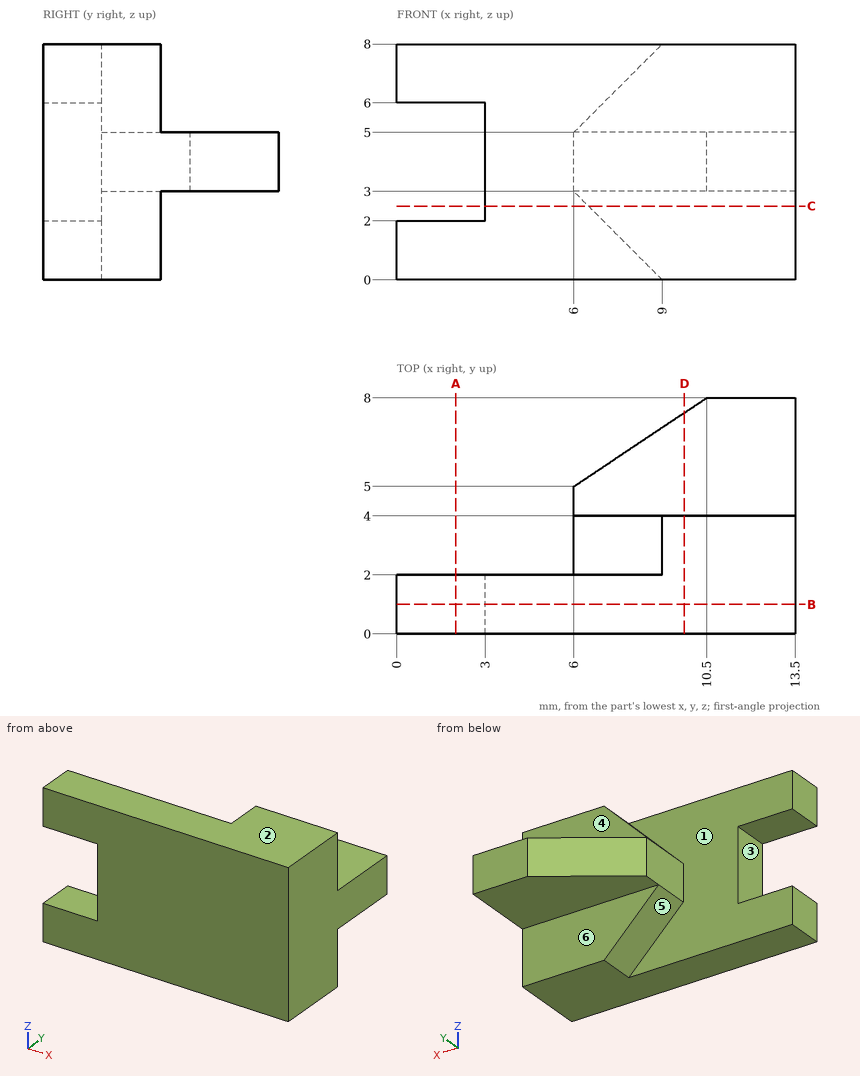
Check sheet for the drawn part. Datum: minimum x, y, z corner. Units: mm. A direction names the side the tool comes from. Give positions to 0.01 mm unless a question says otherwise; leave off trailing zeros. Order: outer loops, then holes, each group sorted by start corner. A loop starts at its lowest first (then second) coordinate and runs counter-clockwise, first axis right, second up. Notation, with made-up numbers: (-38, 68.25) -> (-25, 68.25) arc R29 ccw to (-25, 98.25) -> close; hole circle Ø7 at (85.5, 81). An arc over 180 degrees is marked (long way). One line per item, written item: value.
(1) Tool access check on the marked faces 4, 5 and 6. Record the directions out of +Z, -Z, +X, -X, +Y, -Y that give a thin tool (end or side, any length) a straight path to the whole face; none if there is none.
Final values:
face 4: +Z, +X, -X, +Y
face 5: -Z, -X, +Y
face 6: -Z, +X, -X, +Y
(2) Sectioned sample at A-A on x = 2. Record the cut outline in (y, z).
Final values:
outline: (0, 0) -> (2, 0) -> (2, 2) -> (0, 2) -> close; (0, 6) -> (2, 6) -> (2, 8) -> (0, 8) -> close
(3) Sectioned sample at C-C on z = 2.5. Record the cut outline in (x, y).
Final values:
outline: (3, 0) -> (13.5, 0) -> (13.5, 4) -> (6.5, 4) -> (6.5, 2) -> (3, 2) -> close
(4) Sectioned sample at D-D on x = 9.75. Record the cut outline in (y, z).
Final values:
outline: (0, 0) -> (4, 0) -> (4, 3) -> (7.5, 3) -> (7.5, 5) -> (4, 5) -> (4, 8) -> (0, 8) -> close
(5) Draft check along Z on the marked faces 1, 2 and 3. Enter one of: pulls with the +Z half, pulls with the -Z half, needs draft (parallel to the pull), parting line crosses it, or undercut.
Final values:
face 1: needs draft
face 2: pulls with the +Z half
face 3: undercut
(6) Gauge pin test, flat ends, axial feed: pin 1 (4 mm diameter, centred on x = 6, z = 2.5, fed in from +Y); pin 2 (2 mm diameter, centred on x = 5.5, y = 6, fed in from +Z); pin 3 (2.5 mm diameter, centred on x = 8, z = 6.5, fed in from +Y); pin 4 (0.6 mm diameter, centred on y = 1, z = 4, fed in from -X). Record the tip position at first contact, or that the pin passes through.
Final values:
pin 1: y = 6.29
pin 2: through
pin 3: y = 4
pin 4: x = 3
(7) Scan lines: line 1 along Z through (x, y) = (12.25, 6.5); line 2 along Y through (x, z) = (9.5, 1.75); line 3 along Y through (x, z) = (7.5, 4.5). Record each from-to range of solid material in increasing order. Write a range as [from, to].
Final values:
line 1: [3, 5]
line 2: [0, 4]
line 3: [0, 6]
(8) Sectioned sample at B-B on y = 1. Record the cut outline in (x, z).
Final values:
outline: (0, 0) -> (13.5, 0) -> (13.5, 8) -> (0, 8) -> (0, 6) -> (3, 6) -> (3, 2) -> (0, 2) -> close
